Design review of the part built by this model. Coordinates are the model's own, in mm. Face numbers are marked on the shaded views. A direction names the side the tool comes from. Coordinates: 2 decimals unless noted, no trailing zeros. Write each loop counter-clockwise with the first axis right and the second up, starting at its lowest first coordinate (ties: lowest second). Pieces come first, ordered by that corner, then holes. Notation, with made-up numbers: (33.5, -8) -> (86.5, -8) arc R29 ccw to (86.5, 28) -> close; hole circle Ø1 at (30, 11.25). An arc over 180 degrees is marked (long way). Return JSON: item names as keys, results as strings. Group by question number.
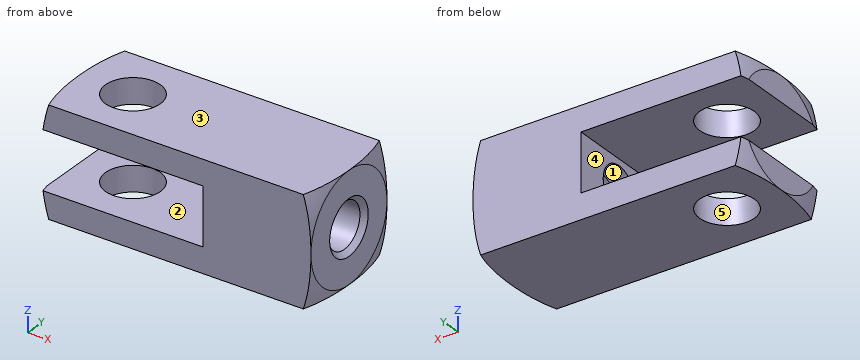
Autodesk Inventor part; units mm, degrees
ref_plane "dummy_XY" through (0, 0, 0) normal (0, 0, 1) x (1, 0, 0)
ref_plane "dummy_YZ" through (0, 0, 0) normal (1, 0, 0) x (0, 1, 0)
ref_plane "dummy_ZX" through (0, 0, 0) normal (0, 1, 0) x (0, 0, 1)
sketch "Sketch_1" plane through (0, 0, 0) normal (0, 0, 1) x (1, 0, 0)
  line L0 (-4.7498, -4.7625) -> (19.05, -4.7625)
  line L1 (19.05, -4.7625) -> (19.05, 4.7625)
  line L2 (19.05, 4.7625) -> (-4.7498, 4.7625)
  line L3 (-4.7498, 4.7625) -> (-4.7498, -4.7625)
extrude "Extrusion1" add sketch "Sketch_1" along normal mid plane 9.525
sketch "Sketch_2" plane through (0, 0, 0) normal (0, 1, 0) x (-1, 0, 0)
  line L0 (4.7498, 2.54) -> (-9.525, 2.54)
  line L1 (-9.525, 2.54) -> (-9.525, -2.54)
  line L2 (-9.525, -2.54) -> (4.7498, -2.54)
  line L3 (4.7498, -2.54) -> (4.7498, 2.54)
extrude "Extrusion2" cut sketch "Sketch_2" along normal mid plane 9.525
sketch "Sketch_3" plane through (0, 0, 0) normal (0, 0, 1) x (1, 0, 0)
  line L0 (19.05, 0) -> (11.176, 0)
  line L1 (11.176, 0) -> (11.176, 1.9837)
  line L2 (11.176, 1.9837) -> (18.6207, 1.9837)
  line L3 (18.6207, 1.9837) -> (19.05, 2.413)
  line L4 (19.05, 2.413) -> (19.05, 0)
  line L5 (19.05, 0) -> (11.176, 0)
revolve "Revolution1" cut sketch "Sketch_3" angle 360 about axis through (19.05, 0, 0) along (1, 0, 0)
sketch "Sketch5" plane through (11.176, 0, 0) normal (1, 0, 0) x (0, 0, -1)
  point P0 (0, 0)
hole "Hole1" at (11.176, 0, 0) direction (-1, 0, 0) diameter 3.9675 depth 1.651
sketch "Sketch6" plane through (0, 0, -4.7625) normal (0, 0, -1) x (-1, 0, 0)
  point P0 (0, 0)
hole "Hole2" at (0, 0, -4.7625) direction (0, 0, 1) diameter 4.826 depth 9.525
sketch "Sketch_9" plane through (0, 0, 0) normal (0, 0, 1) x (1, 0, 0)
  line L0 (23.8125, 0) -> (19.05, 0)
  line L1 (19.05, 0) -> (19.05, 4.7625)
  arc A0 (19.05, 4.7625) -> (16.51, 9.525) centre (8.8503, 2.3812) ccw
  line L2 (16.51, 9.525) -> (23.8125, 9.525)
  line L3 (23.8125, 9.525) -> (23.8125, 0)
  line L4 (23.8125, 0) -> (19.05, 0)
revolve "Revolution2" cut sketch "Sketch_9" angle 360 about axis through (23.8125, 0, 0) along (1, 0, 0)
sketch "Sketch_10" plane through (0, 0, 0) normal (0, 0, 1) x (1, 0, 0)
  line L0 (-4.7498, 0) -> (-9.5123, 0)
  line L1 (-9.5123, 0) -> (-9.5123, 9.525)
  line L2 (-9.5123, 9.525) -> (-2.2098, 9.525)
  arc A0 (-2.2098, 9.525) -> (-4.7498, 4.7625) centre (5.4499, 2.3813) ccw
  line L3 (-4.7498, 4.7625) -> (-4.7498, 0)
  line L4 (-4.7498, 0) -> (-9.5123, 0)
revolve "Revolution3" cut sketch "Sketch_10" angle 360 about axis through (-4.7498, 0, 0) along (1, 0, 0)
ref_plane "dummy_XY" through (0, 0, 0) normal (0, 0, 1) x (1, 0, 0)
ref_plane "dummy_YZ" through (0, 0, 0) normal (1, 0, 0) x (0, 1, 0)
ref_plane "dummy_ZX" through (0, 0, 0) normal (0, 1, 0) x (0, 0, 1)
ref_plane "h1_XY" through (-4.7498, 4.7625, 0) normal (0, 0, 1) x (1, 0, 0)
ref_plane "h1_YZ" through (-4.7498, 4.7625, 0) normal (1, 0, 0) x (0, 1, 0)
ref_plane "h1_ZX" through (-4.7498, 4.7625, 0) normal (0, 1, 0) x (0, 0, 1)
ref_plane "h2_XY" through (-4.7498, -4.7625, 0) normal (0, 0, 1) x (1, 0, 0)
ref_plane "h2_YZ" through (-4.7498, -4.7625, 0) normal (1, 0, 0) x (0, 1, 0)
ref_plane "h2_ZX" through (-4.7498, -4.7625, 0) normal (0, 1, 0) x (0, 0, 1)
ref_plane "l1_XY" through (19.05, 4.7625, 0) normal (0, 0, 1) x (1, 0, 0)
ref_plane "l1_YZ" through (19.05, 4.7625, 0) normal (1, 0, 0) x (0, 1, 0)
ref_plane "l1_ZX" through (19.05, 4.7625, 0) normal (0, 1, 0) x (0, 0, 1)
ref_plane "l11_XY" through (19.05, 4.7625, 0) normal (0, 0, 1) x (1, 0, 0)
ref_plane "l11_YZ" through (19.05, 4.7625, 0) normal (1, 0, 0) x (0, 1, 0)
ref_plane "l11_ZX" through (19.05, 4.7625, 0) normal (0, 1, 0) x (0, 0, 1)
ref_plane "l12_XY" through (0, 4.7625, 0) normal (0, 0, 1) x (1, 0, 0)
ref_plane "l12_YZ" through (0, 4.7625, 0) normal (1, 0, 0) x (0, 1, 0)
ref_plane "l12_ZX" through (0, 4.7625, 0) normal (0, 1, 0) x (0, 0, 1)
ref_plane "l2_XY" through (-4.7498, 4.7625, 0) normal (0, 0, 1) x (1, 0, 0)
ref_plane "l2_YZ" through (-4.7498, 4.7625, 0) normal (1, 0, 0) x (0, 1, 0)
ref_plane "l2_ZX" through (-4.7498, 4.7625, 0) normal (0, 1, 0) x (0, 0, 1)
ref_plane "l21_XY" through (19.05, 0, 0) normal (0, 1, 0) x (1, 0, 0)
ref_plane "l21_YZ" through (19.05, 0, 0) normal (1, 0, 0) x (0, 0, -1)
ref_plane "l21_ZX" through (19.05, 0, 0) normal (0, 0, -1) x (0, 1, 0)
ref_plane "l22_XY" through (9.525, 0, 0) normal (0, 1, 0) x (1, 0, 0)
ref_plane "l22_YZ" through (9.525, 0, 0) normal (1, 0, 0) x (0, 0, -1)
ref_plane "l22_ZX" through (9.525, 0, 0) normal (0, 0, -1) x (0, 1, 0)
ref_plane "piston_rod_clevis_XY" through (19.05, 0, 0) normal (1, 0, 0) x (0, 0, -1)
ref_plane "piston_rod_clevis_YZ" through (19.05, 0, 0) normal (0, 0, -1) x (0, 1, 0)
ref_plane "piston_rod_clevis_ZX" through (19.05, 0, 0) normal (0, 1, 0) x (1, 0, 0)
ref_plane "rod_clevis_body_XY" through (0, 0, 0) normal (0, 0, 1) x (1, 0, 0)
ref_plane "rod_clevis_body_YZ" through (0, 0, 0) normal (1, 0, 0) x (0, 1, 0)
ref_plane "rod_clevis_body_ZX" through (0, 0, 0) normal (0, 1, 0) x (0, 0, 1)
ref_plane "th1_XY" through (19.05, 2.413, 0) normal (0, 0, 1) x (1, 0, 0)
ref_plane "th1_YZ" through (19.05, 2.413, 0) normal (1, 0, 0) x (0, 1, 0)
ref_plane "th1_ZX" through (19.05, 2.413, 0) normal (0, 1, 0) x (0, 0, 1)
ref_plane "th2_XY" through (19.05, -2.413, 0) normal (0, 0, 1) x (1, 0, 0)
ref_plane "th2_YZ" through (19.05, -2.413, 0) normal (1, 0, 0) x (0, 1, 0)
ref_plane "th2_ZX" through (19.05, -2.413, 0) normal (0, 1, 0) x (0, 0, 1)
ref_plane "to_cylinder_XY" through (9.525, 0, 0) normal (1, 0, 0) x (0, 0, -1)
ref_plane "to_cylinder_YZ" through (9.525, 0, 0) normal (0, 0, -1) x (0, 1, 0)
ref_plane "to_cylinder_ZX" through (9.525, 0, 0) normal (0, 1, 0) x (1, 0, 0)
ref_plane "w1_XY" through (19.05, 0, -4.7625) normal (0, 1, 0) x (1, 0, 0)
ref_plane "w1_YZ" through (19.05, 0, -4.7625) normal (1, 0, 0) x (0, 0, -1)
ref_plane "w1_ZX" through (19.05, 0, -4.7625) normal (0, 0, -1) x (0, 1, 0)
ref_plane "w11_XY" through (-4.7498, 0, -2.54) normal (0, 1, 0) x (1, 0, 0)
ref_plane "w11_YZ" through (-4.7498, 0, -2.54) normal (1, 0, 0) x (0, 0, -1)
ref_plane "w11_ZX" through (-4.7498, 0, -2.54) normal (0, 0, -1) x (0, 1, 0)
ref_plane "w12_XY" through (-4.7498, 0, 2.54) normal (0, 1, 0) x (1, 0, 0)
ref_plane "w12_YZ" through (-4.7498, 0, 2.54) normal (1, 0, 0) x (0, 0, -1)
ref_plane "w12_ZX" through (-4.7498, 0, 2.54) normal (0, 0, -1) x (0, 1, 0)
ref_plane "w2_XY" through (19.05, 0, 4.7625) normal (0, 1, 0) x (1, 0, 0)
ref_plane "w2_YZ" through (19.05, 0, 4.7625) normal (1, 0, 0) x (0, 0, -1)
ref_plane "w2_ZX" through (19.05, 0, 4.7625) normal (0, 0, -1) x (0, 1, 0)
properties part number "D-14043"
Q1. Wall thickness on L1, parallel to Z at x = 8, y = 4; L2, parallel to X at y = 0, z = -3.55; L3, parallel to Y at x = 0, z = -3.65: over which ranges is each line inside the solid? List them lowest first.
Q2. For P1, Ø4, axis at y = 2, z = 0, coming from the -X side (3 decimals); P2, Ø3, axis at x = 0, y = 0, coming from the -Z side, all flat-tipped, find the tip position at first contact; note any pin that passes through.
Q3. We need section A-A on x = 0. Write out the cut boundary in (y, z).
Q4. We need section B-B on x = 13. Write out the cut boundary in (y, z), plus the area to 3 significant figures.
Q5. The part is to be moulded in two halves that separate along X. For the marked faces 3, 4 and 5, say which applies: +X half, -X half, draft (parallel to the pull), parting line (faces both ways), or undercut.
Q6. For the marked faces 1 and 2, list the 3-axis set-ups (+Z, -Z, +X, -X, +Y, -Y) from which the entire face can be reached by the end or side of a thin tool; tool diameter is ignored.
Findings below:
{
 "1": {"L1": "z = -4.76 to -2.54, 2.54 to 4.76", "L2": "x = -4.75 to -2.41, 2.41 to 19.05", "L3": "y = -4.76 to -2.41, 2.41 to 4.76"},
 "2": {"P1": "stops at x = 9.525", "P2": "passes through"},
 "3": {"outline": "(-4.76, -4.76) -> (-2.41, -4.76) -> (-2.41, -2.54) -> (-4.76, -2.54) -> close; (-4.76, 2.54) -> (-2.41, 2.54) -> (-2.41, 4.76) -> (-4.76, 4.76) -> close; (2.41, -4.76) -> (4.76, -4.76) -> (4.76, -2.54) -> (2.41, -2.54) -> close; (2.41, 2.54) -> (4.76, 2.54) -> (4.76, 4.76) -> (2.41, 4.76) -> close"},
 "4": {"outline": "(-4.76, -4.76) -> (4.76, -4.76) -> (4.76, 4.76) -> (-4.76, 4.76) -> close; hole circle Ø3.97 at (0, 0)", "area": "78.4 mm^2"},
 "5": {"face 3": "draft", "face 4": "-X half", "face 5": "undercut"},
 "6": {"face 1": "+X, -X", "face 2": "-X, +Y, -Y"}
}
